from build123d import *

# Parameters (mm, degrees)
F0_W     = 25.4
F0_H     = 12.7
F1_DEPTH = 25.4
F2_W     = 6.35
F2_H     = 9.525
F3_DEPTH = 25.4
F5_DEPTH = 25.401


with BuildPart() as f1:
    # F0 (on Front) → F1 (new body)
    with BuildSketch(Plane.XZ):
        Rectangle(F0_W, F0_H)
    extrude(amount=F1_DEPTH)

    # F2 (on face) → F3 (cut)
    with BuildSketch(Plane.XZ.offset(25.4)):
        Rectangle(F2_W, F2_H)
    extrude(amount=-F3_DEPTH, mode=Mode.SUBTRACT)

    # F4 (on face) → F5 (cut, through all)
    with BuildSketch(Plane.XZ.offset(25.4)):
        Polygon((-4.7625, 4.7625), (-3.175, 4.7625), (3.175, 4.7625), (4.7625, 4.7625), (6.35, -3.175), (9.525, -3.175), (9.525, 6.35), (0, 6.35), (-9.525, 6.35), (-9.525, -3.175), (-6.35, -3.175), align=None)
    extrude(amount=-F5_DEPTH, mode=Mode.SUBTRACT)


solid = f1.part
Here's how the part is built. I have some questions about the finished solid (model axes, mm). A direction names the side the tool comes from. Coordinates: 2 decimals unless noted, no trailing zeros. Loops run counter-clockwise (first coordinate to the right, second up) from the corner with the lowest first, then second, coordinate; pieces in that order, holes last.
1. Imagine slicing it at B-B, the plane z = 1. Please give me the cut outline in (x, y) (3 decimals), and give its area (3 significant figures).
2. If we mould it in two halves opening along X, with no side actions, what happens to faces 3 (the flat face through (12.7, -13, 0)), 4 (the flat face through (0, 0, -6)), 5 (the flat face through (3.175, -13, 0))? For each: pulls with the +X half, pulls with the -X half, needs draft (parallel to the pull), parting line crosses it, or undercut.
3. I need wall thicknesses on L1, parallel to X at y = -17.25, z = -4.25 (3 decimals); L2, parallel to X at y = -15, z = 0.25 (3 decimals); L3, parallel to X at y = -7.25, z = -0.75 (3 decimals). Which ranges of each line are inside material? Lowest first, please.
4. For faces 1 (the flat face through (-11, -13, 6.35)), 2 (the flat face through (4, -13, 4.762)), which set-ups out of +Z, -Z, +X, -X, +Y, -Y let a thin tool reach every point of the face, with its end or its side?
5. Imagine slicing it at D-D, the plane x = 1. Please give me the cut outline in (y, z).
6. For P1, Ø1.6, axis at x = -7.5, y = -18, coming from the +Z side (3 decimals); P2, Ø3, axis at x = 0, y = -9, coming from the +Z side; P3, Ø0.8, axis at x = -4, y = -13, coming from the +Z side, each with a flat end and sliding along its axis, tell me the tip position at first contact or that it passes through.
7. Imagine slicing it at A-A, the plane z = 5.25. Please give me the cut outline in (x, y) (3 decimals).
Taken from the geometry:
1. outline: (-12.7, -25.4) - (-9.525, -25.4) - (-9.525, 0) - (-12.7, 0) - close; (-5.515, -25.4) - (-3.175, -25.4) - (-3.175, 0) - (-5.515, 0) - close; (3.175, -25.4) - (5.515, -25.4) - (5.515, 0) - (3.175, 0) - close; (9.525, -25.4) - (12.7, -25.4) - (12.7, 0) - (9.525, 0) - close
1. area: 280 mm2
2. face 3: pulls with the +X half
2. face 4: needs draft
2. face 5: undercut
3. L1: x = -12.7 to -3.175, 3.175 to 12.7
3. L2: x = -12.7 to -9.525, -5.665 to -3.175, 3.175 to 5.665, 9.525 to 12.7
3. L3: x = -12.7 to -9.525, -5.865 to -3.175, 3.175 to 5.865, 9.525 to 12.7
4. face 1: +Z, +X, -X, +Y, -Y
4. face 2: +Z, +Y, -Y
5. outline: (-25.4, -6.35) - (0, -6.35) - (0, -4.76) - (-25.4, -4.76) - close
6. P1: stops at z = -3.175
6. P2: stops at z = -4.76
6. P3: stops at z = 4.76
7. outline: (-12.7, -25.4) - (-9.525, -25.4) - (-9.525, 0) - (-12.7, 0) - close; (9.525, -25.4) - (12.7, -25.4) - (12.7, 0) - (9.525, 0) - close
